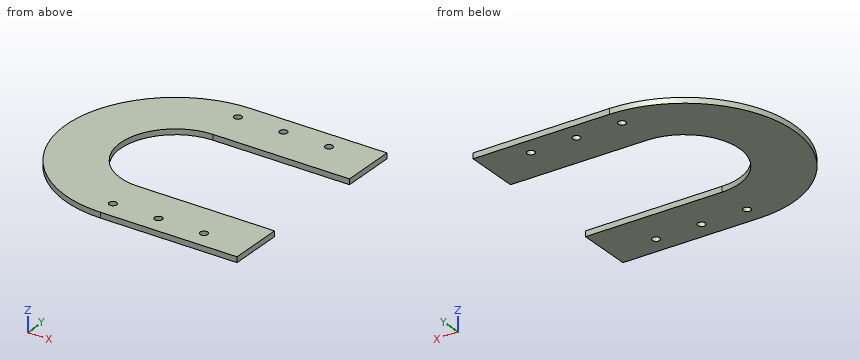
Autodesk Fusion 360 part; units mm, degrees
sketch "草图1" plane through (0, 0, 0) normal (0, 0, 1) x (1, 0, 0)
  line L0 (0, 60) -> (75, 60)
  line L1 (75, 60) -> (75, 30)
  line L2 (75, 30) -> (0, 30)
  line L3 (0, -60) -> (75, -60)
  line L4 (75, -60) -> (75, -30)
  line L5 (75, -30) -> (0, -30)
  arc A0 (0, 60) -> (0, -60) centre (0, 0) ccw
  arc A1 (0, 30) -> (0, -30) centre (0, 0) ccw
  circle A2 centre (0, 50) radius 2.1
  circle A3 centre (25, 50) radius 2.1
  circle A4 centre (50, 50) radius 2.1
  circle A5 centre (0, -50) radius 2.1
  circle A6 centre (25, -50) radius 2.1
  circle A7 centre (50, -50) radius 2.1
  dimension "d1" = 4.2
  dimension "d2" = 4.2
  dimension "d3" = 4.2
  dimension "d4" = 4.2
  dimension "d5" = 4.2
  dimension "d6" = 4.2
extrude "拉伸1" add sketch "草图1" along normal blind 3
sketch "草图2" plane through (0, 0, 0) normal (0, 1, 0) x (1, 0, 0)
sketch "草图3" plane through (0, 0, 0) normal (0, 0, 1) x (1, 0, 0)
Build history of the part. All positions in model axes, mm. Give positions to 0.01 mm unless a question says otherwise; leave off trailing zeros. Order: outer loops, then holes, each group sorted by start corner. A loop starts at its lowest first (then second) coordinate and runs counter-clockwise, first axis right, second up. Notation, with made-up numbers: M 50.5,-7 L 81.5,-7 A23 ccw 81.5,22 Z; hole C -2,59 d10. An arc over 180 degrees is marked long. Return JSON: item names as keys, results as strings.
Q1. Flat gauge pins, fed straight in: pin 1 (1.5 mm diameter, centred on x = -31, z = 0.5, fed in from -Y); pin 2 (1 mm diameter, centred on x = -36, z = 0.5, fed in from -Y). Where does each tip first touch, or does it go through?
Answer list:
{"pin 1": "stops at y = -51.82", "pin 2": "stops at y = -48.37"}
Q2. Wall check: probe 1 along Y at (x, z) = (50, 1.85); probe 2 along Y at (x, z) = (65.5, 1.25); probe 3 along Y at (x, z) = (1, 0.45). Give the ranges that are in metal, low to high. Write a range as from..to.
Answer list:
{"probe 1": "y = -60..-52.1, -47.9..-30, 30..47.9, 52.1..60", "probe 2": "y = -60..-30, 30..60", "probe 3": "y = -60..-51.85, -48.15..-30, 30..48.15, 51.85..60"}
Q3. Band-saw the part on B-B (z = 1.8). Give the cut face in (x, y), then the cut area to 3 significant figures.
Answer list:
{"outline": "M 0,-60 L 75,-60 L 75,-30 L 0,-30 A30 cw 0,30 L 75,30 L 75,60 L 0,60 A60 ccw Z; hole C 0,-50 d4.2; hole C 0,50 d4.2; hole C 25,-50 d4.2; hole C 25,50 d4.2; hole C 50,-50 d4.2; hole C 50,50 d4.2", "area": "8,660 mm^2"}
Q4. Band-saw the part on A-A (x = 50). Give the cut face in (y, z).
Answer list:
{"outline": "M -60,0 L -52.1,0 L -52.1,3 L -60,3 Z; M -47.9,0 L -30,0 L -30,3 L -47.9,3 Z; M 30,0 L 47.9,0 L 47.9,3 L 30,3 Z; M 52.1,0 L 60,0 L 60,3 L 52.1,3 Z"}
Q5. Band-saw the part on D-D (x = -48). Give the cut face in (y, z).
Answer list:
{"outline": "M -36,0 L 36,0 L 36,3 L -36,3 Z"}
Q6. Band-saw the part on C-C (y = 50). Give the cut face in (x, z).
Answer list:
{"outline": "M -33.17,0 L -2.1,0 L -2.1,3 L -33.17,3 Z; M 2.1,0 L 22.9,0 L 22.9,3 L 2.1,3 Z; M 27.1,0 L 47.9,0 L 47.9,3 L 27.1,3 Z; M 52.1,0 L 75,0 L 75,3 L 52.1,3 Z"}
